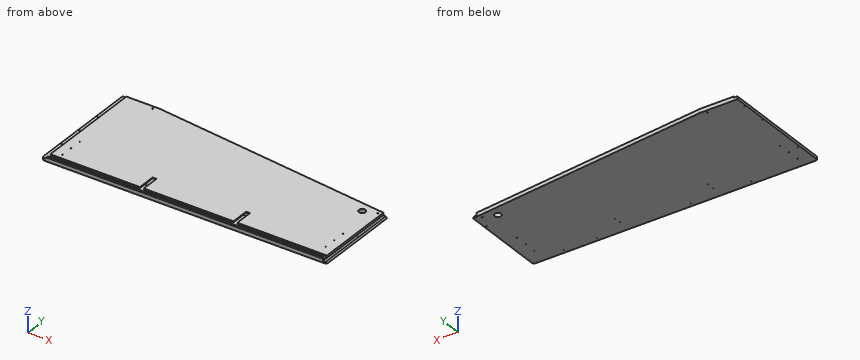
from build123d import *

# Parameters (mm, degrees)
EXTRUDE2_DEPTH     = 17.78
CUT_EXTRUDE3_DEPTH = 5.08
SKETCH9_R          = 3.174999999
CUT_EXTRUDE4_DEPTH = 5.08
SKETCH10_R         = 15.08125
SKETCH10_R_2       = 2.36855
SKETCH10_R_3       = 1.5875
CUT_EXTRUDE5_DEPTH = 17.78
SKETCH11_W         = 25.7175
SKETCH11_H         = 413.5501
CUT_EXTRUDE6_DEPTH = 11.43
CUT_EXTRUDE8_REACH = 10238.765


with BuildPart() as part:
    # Sketch7 → Extrude2 (new body)
    with BuildSketch(Plane.XY):
        Polygon((9086.320833334, -4722.091838581), (10222.970833334, -4853.78125), (10222.970833334, -5248.275), (10218.208333334, -5253.0375), (8919.633333334, -5253.0375), (8914.870833334, -5248.275), (8914.870833334, -4722.091838581), align=None)
    extrude(amount=-EXTRUDE2_DEPTH)

    # Sketch8 → Cut-Extrude3 (cut)
    with BuildSketch(Plane.XY):
        Polygon((8932.650833334, -4715.591300541), (8911.695833334, -4715.591300541), (8911.695833334, -5256.2125), (8932.650833334, -5256.2125), (8932.650833334, -5243.5125), (10226.145833334, -5243.5125), (10226.145833334, -5225.7325), (9792.864166667, -5225.7325), (9792.864166667, -5146.402628061), (9788.374038608, -5141.912499999), (9779.574294729, -5141.912499999), (9775.084166668, -5146.402628059), (9775.084166668, -5225.7325), (9362.757500002, -5225.7325), (9362.757500002, -5146.402628059), (9358.267371941, -5141.9125), (9349.467628062, -5141.9125), (9344.9775, -5146.402628059), (9344.9775, -5225.7325), (8932.650833334, -5225.7325), align=None)
    extrude(amount=-CUT_EXTRUDE3_DEPTH, mode=Mode.SUBTRACT)

    # Sketch9 → Cut-Extrude4 (cut)
    with BuildSketch(Plane.XY):
        with Locations((9347.22256403, -5144.157564029)):
            Circle(SKETCH9_R)
        with Locations((9360.512435972, -5144.157564029)):
            Circle(SKETCH9_R)
        with Locations((9777.329230699, -5144.157564029)):
            Circle(SKETCH9_R)
        with Locations((9790.619102638, -5144.157564029)):
            Circle(SKETCH9_R)
    extrude(amount=-CUT_EXTRUDE4_DEPTH, mode=Mode.SUBTRACT)

    # Sketch10 → Cut-Extrude5 (cut)
    with BuildSketch(Plane.XY):
        with Locations((10132.081036572, -4887.549352662)):
            Circle(SKETCH10_R)
        with Locations((9062.659822767, -4736.376540025)):
            Circle(SKETCH10_R_2)
        with Locations((8923.760833334, -4778.904166666)):
            Circle(SKETCH10_R_3)
        with Locations((8923.760833334, -4897.4375)):
            Circle(SKETCH10_R_3)
        with Locations((8923.760833334, -5015.970833334)):
            Circle(SKETCH10_R_3)
        with Locations((8923.760833334, -5134.504166666)):
            Circle(SKETCH10_R_3)
        with Locations((9054.570833334, -5234.6225)):
            Circle(SKETCH10_R_3)
        with Locations((9206.970833334, -5234.6225)):
            Circle(SKETCH10_R_3)
        with Locations((9353.8675, -5193.9825)):
            Circle(SKETCH10_R_3)
        with Locations((9353.8675, -5160.9625)):
            Circle(SKETCH10_R_3)
        with Locations((9486.370833334, -5234.6225)):
            Circle(SKETCH10_R_3)
        with Locations((9638.770833334, -5234.6225)):
            Circle(SKETCH10_R_3)
        with Locations((9783.974166666, -5193.9825)):
            Circle(SKETCH10_R_3)
        with Locations((9783.974166666, -5160.9625)):
            Circle(SKETCH10_R_3)
        with Locations((9918.170833334, -5234.6225)):
            Circle(SKETCH10_R_3)
        with Locations((10070.570833334, -5234.6225)):
            Circle(SKETCH10_R_3)
        with Locations((10214.080833334, -5031.58125)):
            Circle(SKETCH10_R_3)
        with Locations((10214.080833334, -4929.98125)):
            Circle(SKETCH10_R_3)
        with Locations((10190.180218809, -4867.008218481)):
            Circle(SKETCH10_R_2)
        with Locations((8972.338333334, -5087.9375)):
            Circle(SKETCH10_R_3)
        with Locations((8972.338333334, -5145.0875)):
            Circle(SKETCH10_R_3)
        with Locations((8972.338333334, -5202.2375)):
            Circle(SKETCH10_R_3)
        with Locations((10165.503333334, -5176.8375)):
            Circle(SKETCH10_R_3)
        with Locations((10165.503333334, -5119.6875)):
            Circle(SKETCH10_R_3)
        with Locations((10165.503333334, -5062.5375)):
            Circle(SKETCH10_R_3)
    extrude(amount=-CUT_EXTRUDE5_DEPTH, mode=Mode.SUBTRACT)

    # Sketch11 → Cut-Extrude6 (cut)
    with BuildSketch(Plane.XY):
        with Locations((10218.049583334, -5051.02495)):
            Rectangle(SKETCH11_W, SKETCH11_H)
    extrude(amount=-CUT_EXTRUDE6_DEPTH, mode=Mode.SUBTRACT)

    # Cut-Extrude8: up to this plane
    cut_extrude8_end = Plane(origin=(9086.320833334, -4722.091838581, -17.78), z_dir=(0.11508765240352697, 0.993355340381399, 0))
    # Sketch14 → Cut-Extrude8 (cut, up to the surface)
    with BuildSketch(Plane.XZ.offset(5253.0375), mode=Mode.PRIVATE) as cut_extrude8_sk1:
        Polygon((10222.970833334, -11.43), (10229.320833334, -11.43), (10222.970833334, -17.78), (10216.620833334, -11.43), align=None)
    cut_extrude8_tool1 = split(extrude(cut_extrude8_sk1.sketch, amount=-CUT_EXTRUDE8_REACH, mode=Mode.PRIVATE), bisect_by=cut_extrude8_end, keep=Keep.BOTH, mode=Mode.PRIVATE)
    add(cut_extrude8_tool1.solids().sort_by_distance((10222.970833, -5253.0375, -13.546667))[0], mode=Mode.SUBTRACT)


solid = part.part
Geometry check sheet. Reference: the model listing, model coordinates, mm. Round coordinates to 2 decimals unless told otherwise and drop trailing zeros. Write each loop counter-clockwise with the first axis right and the second up, starting at its lowest first coordinate (ties: lowest second). Pieces come first, ordered by that corner, then holes.
Item 1: Go/stop test with flat-tipped pins: pin 1 Ø10 at (y, z) = (-5016.5, -7) entering from +X; pin 2 Ø3.5 at (x, y) = (10214.08, -5031.58) entering from +Z; pin 3 Ø6 at (x, z) = (9984, -14.5) entering from +Y; pin 4 Ø1.9 at (x, y) = (10165.5, -5176.84) entering from +Z. Record where each tip stops, or that it passes through.
Determined:
pin 1: stops at x = 10217.19
pin 2: stops at z = -11.43
pin 3: stops at y = -4825.75
pin 4: passes through
Item 2: Section check D-D (x = 9749.5). Record the boundary of the cut face in (y, z).
Determined:
outline: (-5253.04, -17.78) - (-4798.93, -17.78) - (-4798.93, 0) - (-5225.73, 0) - (-5225.73, -5.08) - (-5243.51, -5.08) - (-5243.51, 0) - (-5253.04, 0) - close
Item 3: Section check C-C (y = -4833.5). Record the boundary of the cut face in (x, z), plus the area to 3 significant figures.
Determined:
outline: (8914.87, -17.78) - (10047.92, -17.78) - (10047.92, 0) - (8932.65, 0) - (8932.65, -5.08) - (8914.87, -5.08) - close
area: 20,100 mm2
Item 4: Material ranges on line 1 along X through (y, z) = (-5047.5, -13); line 2 along Y through (x, z) = (9592, -1.5); line 3 along X through (y, z) = (-5203, -13.5), recorded low to high.
Determined:
line 1: x = 8914.87 to 10218.19
line 2: y = -5253.04 to -5243.51, -5225.73 to -4780.68
line 3: x = 8914.87 to 8970.95, 8973.73 to 10218.69
Item 5: Section check B-B (x = 10000). Record the boundary of the cut face in (y, z), plus the area to 3 significant figures.
Determined:
outline: (-5253.04, -17.78) - (-4827.95, -17.78) - (-4827.95, 0) - (-5225.73, 0) - (-5225.73, -5.08) - (-5243.51, -5.08) - (-5243.51, 0) - (-5253.04, 0) - close
area: 7,470 mm2
Item 6: Section check A-A (z = -8). Give the number of separate pieces and of enclosed holes in the cut face, plus the area to 3 significant figures.
Determined:
separate pieces: 1
enclosed holes: 23
area: 612,000 mm2
